The drawing under review shows one solid part. Ordinate dimensions are in mm from its lowest x, y, z. A direction names the side the tool comes from. Round coordinates to 2 decimals unless told otherwise and drop trailing zeros. Order: outer loops, then holes, each group sorted by start corner. A loop starts at its lowest first (then second) coordinate and runs counter-clockwise, first axis right, second up. Notation, with made-up numbers: (-37, 29.5) -> (-12, 29.5) arc R13 ccw to (-12, 44.5) -> close; hole circle Ø7 at (41.5, -9.5). An arc over 180 degrees is marked (long way). Put each result on its own line as item: value. Start each with the question number.
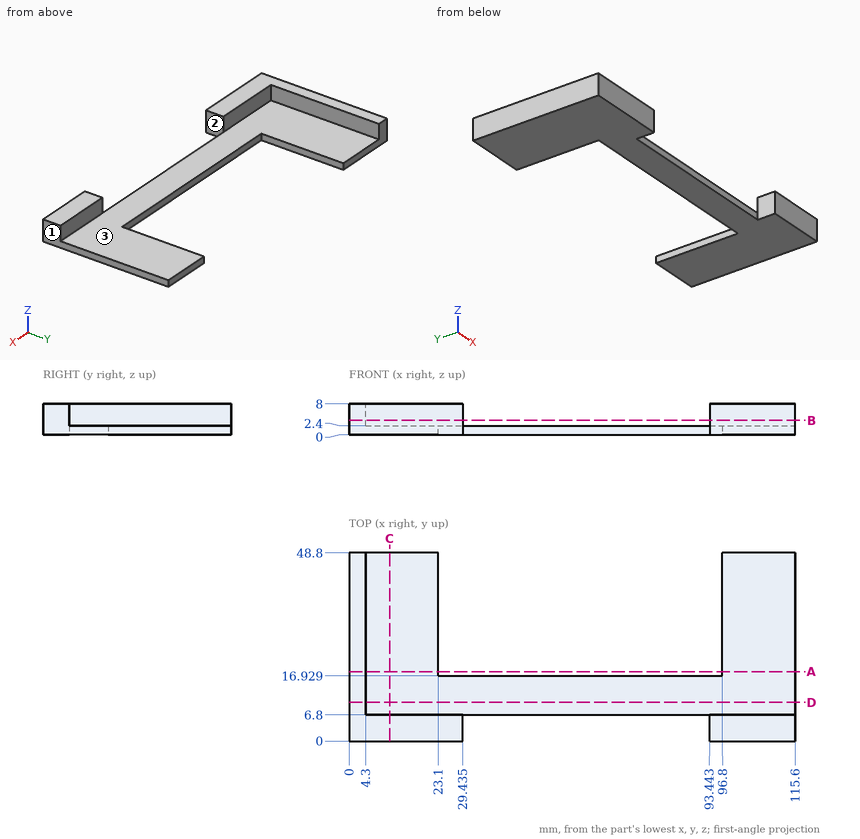
Item 1: Consider section B-B, the plane z = 3.75. Write out the cut boundary in (x, y) (1 decimal).
Item 2: Consider section D-D, the plane y = 10. Write out the cut boundary in (x, z).
Item 3: Tool access review of the marked faces 1, 2 and 3: name each direction out of +Z, -Z, +X, -X, +Y, -Y from which nothing blocks a thin tool from reaching the whole face with its end or side.
Item 4: Consider section C-C, the plane x = 10.5. Write out the cut boundary in (y, z), plus the area to 3 significant figures.
Item 5: Insertion check: pin 1 Ø1.2 at (x, z) = (57.5, 1) entering from -Y; pin 2 Ø21 at (x, y) = (51, 24.5) entering from +Z; pin 3 Ø1.7 at (x, z) = (21, 6) entering from +Y. Each pin has a flat end and moves straight along its axis. Give the tip position at first contact, or say it passes through.
Item 6: For L1, parallel to X at y = 4.5, z = 3.75 (1 decimal); L2, parallel to Z at x = 103, y = 13.5; L3, parallel to X at y = 9.5, z = 5.5, list the stretches that pass through material, from the lowest coordinate up.
Item 7: Consider section A-A, the plane y = 18. Write out the cut boundary in (x, z), plus the area to 3 significant figures.
Evaluation:
1. outline: (0, 0) -> (29.4, 0) -> (29.4, 6.8) -> (4.3, 6.8) -> (4.3, 48.8) -> (0, 48.8) -> close; (93.4, 0) -> (115.6, 0) -> (115.6, 6.8) -> (93.4, 6.8) -> close
2. outline: (0, 0) -> (115.6, 0) -> (115.6, 2.4) -> (4.3, 2.4) -> (4.3, 8) -> (0, 8) -> close
3. face 1: +Z, -Z, +X, +Y, -Y
3. face 2: +Z, -Z, -Y
3. face 3: +Z, +X, +Y
4. outline: (0, 0) -> (48.8, 0) -> (48.8, 2.4) -> (6.8, 2.4) -> (6.8, 8) -> (0, 8) -> close
4. area: 155 mm^2
5. pin 1: stops at y = 6.8
5. pin 2: stops at z = 2.4
5. pin 3: stops at y = 6.8
6. L1: x = 0 to 29.4, 93.4 to 115.6
6. L2: z = 0 to 2.4
6. L3: x = 0 to 4.3
7. outline: (0, 0) -> (23.1, 0) -> (23.1, 2.4) -> (4.3, 2.4) -> (4.3, 8) -> (0, 8) -> close; (96.8, 0) -> (115.6, 0) -> (115.6, 2.4) -> (96.8, 2.4) -> close
7. area: 125 mm^2
